```python
from build123d import *

# Parameters (mm, degrees)
F0_R      = 5
F1_DEPTH  = 200
F0_R_2    = 47.095
F2_DEPTH  = 2
F3_DEPTH  = 4
F1_FACE_R = 5


with BuildPart() as f1:
    # F0 (on Top) → F1 (new body)
    with BuildSketch(Plane.XY):
        Circle(F0_R)
    extrude(amount=F1_DEPTH)

    # F0 (on Top) → F2 (join)
    with BuildSketch(Plane.XY):
        Circle(F0_R_2)
        Circle(F0_R, mode=Mode.SUBTRACT)
    extrude(amount=F2_DEPTH)

    # F0 (on Top) → F3 (join)
    with BuildSketch(Plane.XY):
        Polygon((-32.5393686004, 42.5539186241), (-53.098972618, 7.0813562323), (-42.5539186241, -32.5393686004), (-7.0813562323, -53.098972618), (32.5393686004, -42.5539186241), (53.098972618, -7.0813562323), (42.5539186241, 32.5393686004), (7.0813562323, 53.098972618), align=None)
        Circle(F0_R_2, mode=Mode.SUBTRACT)
    extrude(amount=F3_DEPTH)

    # F1_face (on face) → F6 section 0
    with BuildSketch(Plane.XY.offset(200), mode=Mode.PRIVATE) as f6_s0:
        Circle(F1_FACE_R)
    loft([Vertex(0, 0, 204), f6_s0.sketch])


solid = f1.part
```
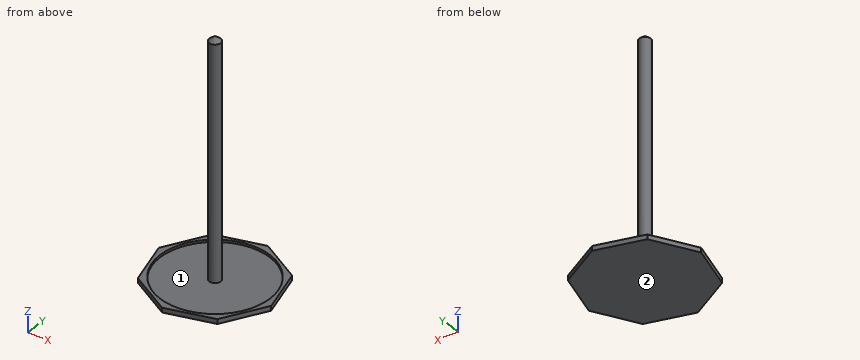
Work out the finished part from the listing and answer in its coordinate system (mm). Face numbers are marked on the shaded views. Round coordinates to 2 decimals unless told otherwise and drop trailing zeros. Write each loop counter-clockwise with the first axis right and the second up, starting at its lowest first coordinate (ties: lowest second). Pieces come first, ordered by that corner, then holes. Notation, with made-up numbers: (-4.5, 5.25) - (18.5, 5.25) arc R22 cw to (18.5, 42.25) - close; hole circle Ø5 at (81.5, -33.75). An arc over 180 degrees is marked (long way). Return JSON: item names as keys, results as strings. Group by question number.
Q1. The mould has two halves that part along Y. Classify the marked faces 1 and 2: released by +Y, released by -Y, zero draft, split by the parting line, or undercut.
Q2. Each of these flat-tipped pins is pushed along its axis until it touches: pin 1 Ø6 at (x, y) = (7, 29) entering from +Z; pin 2 Ø5 at (x, z) = (-3.5, 54) entering from -Y. Where does it stop, or does it pass through?
Q3. The part is cut by section A-A on x = 24. Write down the section's boundary in (y, z).
Q4. Find the intervals of material crossed by L1, parallel to Y at x = 0, z = 2.7 (3 decimals); L2, parallel to Z at x = 5.5, y = 3; L3, parallel to Z at x = 2.5, y = -48, in increasing order.
Q5. The part is cut by section B-B on z = 20.5. Write down the section's boundary in (x, y).
Q6. The part is cut by section C-C on y = 29.5. Write down the section's boundary in (x, z), then the cut area to 3 significant figures.
Solved:
{
 "1": {"face 1": "undercut", "face 2": "zero draft"},
 "2": {"pin 1": "z = 2", "pin 2": "y = -4.9"},
 "3": {"outline": "(-44.83, 0) - (43.29, 0) - (43.29, 4) - (40.52, 4) - (40.52, 2) - (-40.52, 2) - (-40.52, 4) - (-44.83, 4) - close"},
 "4": {"L1": "-51.214 to -47.095, -5 to 5, 47.095 to 51.214", "L2": "0 to 2", "L3": "0 to 4"},
 "5": {"outline": "circle Ø10 at (0, 0)"},
 "6": {"outline": "(-40.11, 0) - (43.36, 0) - (43.36, 4) - (36.71, 4) - (36.71, 2) - (-36.71, 2) - (-36.71, 4) - (-40.11, 4) - close", "area": "187 mm²"}
}
